from build123d import *

# Parameters (mm, degrees)
SKETCH1_W            = 279.4
SKETCH1_H            = 101.6
BOSS_EXTRUDE1_DEPTH  = 6.35
SKETCH2_R            = 13.97
BOSS_EXTRUDE3_DEPTH  = 5.55625
SKETCH9_R            = 11.1125
CUT_EXTRUDE4_DEPTH   = 4.445
CUT_EXTRUDE5_START   = -5.55625
SKETCH10_R           = 11.1125
CUT_EXTRUDE5_DEPTH   = 5.55625
SKETCH11_R           = 7.9375
CUT_EXTRUDE6_DEPTH   = 285.078633923
SKETCH12_R           = 12.7
CUT_EXTRUDE7_DEPTH   = 285.051619429
SKETCH22_W           = 63.5
SKETCH22_H           = 63.5
BOSS_EXTRUDE7_DEPTH  = 12.7
SKETCH25_W           = 50.8
SKETCH25_H           = 50.8
CUT_EXTRUDE11_DEPTH  = 15.875
SKETCH32_R           = 4.7625
CUT_EXTRUDE12_DEPTH  = 6.35
SKETCH38_W           = 46.99
SKETCH38_H           = 18.470251096
CUT_EXTRUDE13_DEPTH  = 6.35
SKETCH50_W           = 49.2899954
SKETCH50_H           = 29.09000024
BOSS_EXTRUDE14_DEPTH = 25.4
SKETCH49_W           = 40.3999954
SKETCH49_H           = 20.20000024
CUT_EXTRUDE19_DEPTH  = 286.114292872
SKETCH52_W           = 20.20000024
SKETCH52_H           = 25.4
CUT_EXTRUDE20_DEPTH  = 4.445
SKETCH53_W           = 44.8449954
SKETCH53_H           = 20.20000024
BOSS_EXTRUDE15_DEPTH = 4.760622178
SKETCH55_W           = 44.8449954
SKETCH55_H           = 20.20000024
CUT_EXTRUDE21_DEPTH  = 285.729668136
SKETCH56_W           = 13.97
SKETCH56_H           = 20.20000024
BOSS_EXTRUDE16_DEPTH = 6.35


with BuildPart() as part:
    # Sketch1 → Boss-Extrude1 (new body)
    with BuildSketch(Plane(origin=(0, 0, 0), x_dir=(1, 0, 0), z_dir=(0, 1, 0))):
        with Locations((-139.7, 0)):
            Rectangle(SKETCH1_W, SKETCH1_H)
    extrude(amount=BOSS_EXTRUDE1_DEPTH)

    # Sketch2 → Boss-Extrude3 (add)
    with BuildSketch(Plane(origin=(0, 6.35, 0), x_dir=(1, 0, 0), z_dir=(0, 1, 0))):
        with Locations(Location((-258.510557857, 0, 0), (0, 0, 90))):
            Circle(SKETCH2_R)
    extrude(amount=BOSS_EXTRUDE3_DEPTH)

    # Sketch9 → Cut-Extrude4 (cut)
    with BuildSketch(Plane(origin=(0, 11.90625, 0), x_dir=(1, 0, 0), z_dir=(0, 1, 0))):
        with Locations(Location((-258.510557857, 0, 0), (0, 0, 270))):
            Circle(SKETCH9_R)
    extrude(amount=-CUT_EXTRUDE4_DEPTH, mode=Mode.SUBTRACT)

    # Sketch10 → Cut-Extrude5 (cut)
    with BuildSketch(Plane(origin=(0, 0, 0), x_dir=(-1, 0, 0), z_dir=(0, -1, 0)).offset(CUT_EXTRUDE5_START)):
        with Locations(Location((258.510557857, 0, 0), (0, 0, 270))):
            Circle(SKETCH10_R)
    extrude(amount=CUT_EXTRUDE5_DEPTH, mode=Mode.SUBTRACT)

    # Sketch11 → Cut-Extrude6 (cut, through all)
    with BuildSketch(Plane(origin=(0, 7.46125, 0), x_dir=(1, 0, 0), z_dir=(0, 1, 0))):
        with Locations(Location((-258.510557857, 0, 0), (0, 0, 270))):
            Circle(SKETCH11_R)
    extrude(amount=-CUT_EXTRUDE6_DEPTH, mode=Mode.SUBTRACT)

    # Sketch12 → Cut-Extrude7 (cut, through all)
    with BuildSketch(Plane(origin=(0, 6.35, 0), x_dir=(1, 0, 0), z_dir=(0, 1, 0))):
        with Locations(Location((-134.666203771, 0, 0), (0, 0, 270))):
            Circle(SKETCH12_R)
    extrude(amount=-CUT_EXTRUDE7_DEPTH, mode=Mode.SUBTRACT)

    # Sketch22 → Boss-Extrude7 (add)
    with BuildSketch(Plane(origin=(0, 6.35, 0), x_dir=(1, 0, 0), z_dir=(0, 1, 0))):
        with Locations((-134.666203771, 0)):
            Rectangle(SKETCH22_W, SKETCH22_H)
    extrude(amount=BOSS_EXTRUDE7_DEPTH)

    # Sketch25 → Cut-Extrude11 (cut)
    with BuildSketch(Plane(origin=(0, 19.05, 0), x_dir=(1, 0, 0), z_dir=(0, 1, 0))):
        with Locations((-134.666203771, 0)):
            Rectangle(SKETCH25_W, SKETCH25_H)
    extrude(amount=-CUT_EXTRUDE11_DEPTH, mode=Mode.SUBTRACT)

    # Sketch32 → Cut-Extrude12 (cut)
    with BuildSketch(Plane(origin=(0, 6.35, 0), x_dir=(1, 0, 0), z_dir=(0, 1, 0))):
        with Locations(Location((-67.44195898, -40.64, 0), (0, 0, 270))):
            Circle(SKETCH32_R)
        with Locations(Location((-81.41195898, -40.64, 0), (0, 0, 270))):
            Circle(SKETCH32_R)
        with Locations(Location((-67.44195898, 40.64, 0), (0, 0, 270))):
            Circle(SKETCH32_R)
        with Locations(Location((-81.41195898, 40.64, 0), (0, 0, 270))):
            Circle(SKETCH32_R)
    extrude(amount=-CUT_EXTRUDE12_DEPTH, mode=Mode.SUBTRACT)

    # Sketch38 → Cut-Extrude13 (cut)
    with BuildSketch(Plane(origin=(0, 6.35, 0), x_dir=(1, 0, 0), z_dir=(0, 1, 0))):
        with Locations((-23.495, -24.777709652)):
            Rectangle(SKETCH38_W, SKETCH38_H)
    extrude(amount=-CUT_EXTRUDE13_DEPTH, mode=Mode.SUBTRACT)

    # Sketch50 → Boss-Extrude14 (add)
    with BuildSketch(Plane(origin=(0, 6.35, 0), x_dir=(1, 0, 0), z_dir=(0, 1, 0))):
        with Locations((-212.910560157, 0)):
            Rectangle(SKETCH50_W, SKETCH50_H)
    extrude(amount=BOSS_EXTRUDE14_DEPTH)

    # Sketch49 → Cut-Extrude19 (cut, through all)
    with BuildSketch(Plane(origin=(0, 6.35, 0), x_dir=(1, 0, 0), z_dir=(0, 1, 0))):
        with Locations((-212.910560157, 0)):
            Rectangle(SKETCH49_W, SKETCH49_H)
    extrude(amount=CUT_EXTRUDE19_DEPTH, mode=Mode.SUBTRACT)

    # Sketch52 → Cut-Extrude20 (cut)
    with BuildSketch(Plane(origin=(-233.110557857, 0, 0), x_dir=(0, 0, -1), z_dir=(1, 0, 0))):
        with Locations((0, 19.05)):
            Rectangle(SKETCH52_W, SKETCH52_H)
    extrude(amount=-CUT_EXTRUDE20_DEPTH, mode=Mode.SUBTRACT)

    # Sketch53 → Boss-Extrude15 (add)
    with BuildSketch(Plane(origin=(0, 6.35, 0), x_dir=(1, 0, 0), z_dir=(0, 1, 0))):
        with Locations((-215.133060157, 0)):
            Rectangle(SKETCH53_W, SKETCH53_H)
    extrude(amount=BOSS_EXTRUDE15_DEPTH)

    # Sketch55 → Cut-Extrude21 (cut, through all)
    with BuildSketch(Plane(origin=(0, 11.110622178, 0), x_dir=(1, 0, 0), z_dir=(0, 1, 0))):
        with Locations((-215.133060157, 0)):
            Rectangle(SKETCH55_W, SKETCH55_H)
    extrude(amount=-CUT_EXTRUDE21_DEPTH, mode=Mode.SUBTRACT)

    # Sketch56 → Boss-Extrude16 (add)
    with BuildSketch(Plane(origin=(0, 6.35, 0), x_dir=(1, 0, 0), z_dir=(0, 1, 0))):
        with Locations((-214.060557857, 0)):
            Rectangle(SKETCH56_W, SKETCH56_H)
    extrude(amount=-BOSS_EXTRUDE16_DEPTH)


solid = part.part
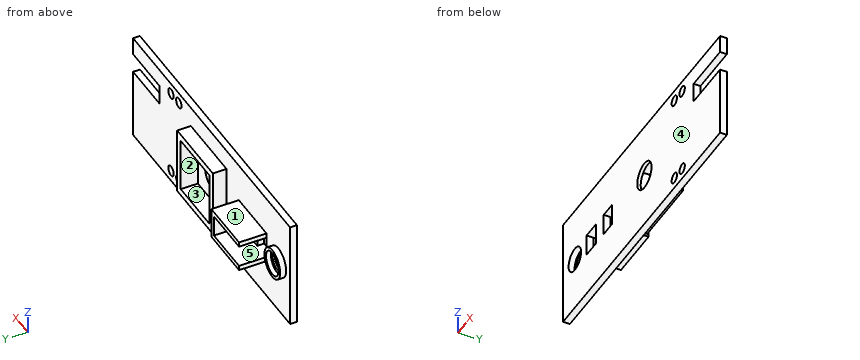
Could you check a few things on this model? Use its own coordinates, in mm. Face numbers are marked on the shaded views. A direction names the side the tool comes from. Give positions to 0.01 mm unless a question says otherwise; leave off trailing zeros. Loops run counter-clockwise (first coordinate to the right, second up) from the corner with the lowest first, then second, coordinate; pieces in that order, holes last. Notation, with made-up numbers: (5.5, 34) -> (52.5, 34) arc R17 cw to (52.5, 53) -> close; hole circle Ø8 at (-21, 33.5). An arc over 180 degrees is marked (long way). Return JSON: item names as keys, results as strings.
Item 1: If we section it at C-C on x = -225: List the corners of the cut face in (y, z) for me (3 decimals), plus the area to 3 significant figures.
Geometry results:
{"outline": "(0, -50.8) -> (6.35, -50.8) -> (6.35, -14.545) -> (31.75, -14.545) -> (31.75, -10.1) -> (0, -10.1) -> close; (0, 10.1) -> (31.75, 10.1) -> (31.75, 14.545) -> (6.35, 14.545) -> (6.35, 50.8) -> (0, 50.8) -> close", "area": "743 mm²"}
Item 2: We'd pull the mould along X, two halves only. Please class the marked faces 1, 2 and 3: +X half, -X half, draft (parallel to the pull), parting line (faces both ways), or undercut.
Geometry results:
{"face 1": "draft", "face 2": "undercut", "face 3": "undercut"}
Item 3: I need wall thicknesses on L1, parallel to X at y = 9.45, z = 0; L2, parallel to X at y = 5, z = -40; L3, parallel to X at y = 6.15, z = 0. Which ranges of each line are inside material? Lowest first, please. Write a range as from..to.
Geometry results:
{"L1": "x = -272.48..-269.62, -247.4..-244.54, -192.71..-188.27, -166.42..-160.07, -109.27..-102.92", "L2": "x = -279.4..-86.13, -76.69..-72.16, -62.72..0", "L3": "x = -279.4..-266.45, -250.57..-237.56, -221.05..-207.08, -192.71..-160.07, -109.27..0"}
Item 4: Which directions (+Z, -Z, +X, -X, +Y, -Y) give clear straight access to the entire face, cutting with the end or side of a thin tool? Please do the marked faces 4 and 5.
Geometry results:
{"face 4": "+Z, -Z, +X, -X, -Y", "face 5": "+Y"}
Item 5: If we section it at B-B on z = 40.64: List the corners of the cut face in (x, y) for me, plus the area to 3 significant figures.
Geometry results:
{"outline": "(-279.4, 0) -> (-86.17, 0) -> (-86.17, 6.35) -> (-279.4, 6.35) -> close; (-76.65, 0) -> (-72.2, 0) -> (-72.2, 6.35) -> (-76.65, 6.35) -> close; (-62.68, 0) -> (0, 0) -> (0, 6.35) -> (-62.68, 6.35) -> close", "area": "1,650 mm²"}
Item 6: If we section it at A-A on x = -18.5: List the corners of the cut face in (y, z) for me.
Geometry results:
{"outline": "(0, -50.8) -> (6.35, -50.8) -> (6.35, 15.54) -> (0, 15.54) -> close; (0, 34.01) -> (6.35, 34.01) -> (6.35, 50.8) -> (0, 50.8) -> close"}
Item 7: If we section it at D-D on z = -21: List the corners of the cut face in (x, y) for me (3 decimals).
Geometry results:
{"outline": "(-279.4, 0) -> (0, 0) -> (0, 6.35) -> (-102.916, 6.35) -> (-102.916, 19.05) -> (-109.266, 19.05) -> (-109.266, 3.175) -> (-160.066, 3.175) -> (-160.066, 19.05) -> (-166.416, 19.05) -> (-166.416, 6.35) -> (-279.4, 6.35) -> close"}
Item 8: I'm going to push flat-ended pins straight in: pin 1 (5 mm diameter, centred on x = -169, y = 19.5, fed in from +Z); pin 2 (8 mm diameter, centred on x = -128, y = 15, fed in from -Z); pin 3 (12.5 mm diameter, centred on x = -127.5, y = 13.5, fed in from +Z); pin 4 (12.5 mm diameter, centred on y = 13.5, z = -1.5, fed in from +X). Where does each tip first touch, or does it pass through?
Geometry results:
{"pin 1": "passes through", "pin 2": "stops at z = -31.75", "pin 3": "stops at z = 31.75", "pin 4": "stops at x = -102.92"}
